Check sheet for the modelled part. Datum: model origin and axes. Units: mm. A direction names the side the tool comes from. Round coordinates to 2 decimals unless told otherwise and drop trailing zeros. Write each loop counter-clockwise with the first axis right and the second up, starting at its lowest first coordinate (ties: lowest second). Pieces come first, ordered by that corner, then holes. Notation, with made-up numbers: M -29.5,44.25 L 1.5,44.25 A14 cw 1.5,56.25 Z; hole C 73.5,31 d9. An arc over 180 degrees is marked long. Put each result on its own line as item: value.
```python
from build123d import *

# Parameters (mm, degrees)
F0_R     = 9.085858
F0_R_2   = 9.713119
F0_R_3   = 9.943087
F1_DEPTH = 20
F0_R_4   = 2.956613
F0_R_5   = 3.792216
F0_R_6   = 3.328406
F2_DEPTH = 10


with BuildPart() as f1:
    # F0 (on Top) → F1 (new body)
    with BuildSketch(Plane.XY):
        with BuildLine():
            ThreePointArc((0, 16), (4.686292, 4.686292), (16, 0))
            Line((16, 0), (62.072559, 0))
            ThreePointArc((62.072559, 0), (77.309287, 11.117161), (71.37237, 29.019736))
            Line((71.37237, 29.019736), (25.299811, 61.928706))
            ThreePointArc((25.299811, 61.928706), (8.678695, 63.135653), (0, 48.908971))
            Line((0, 48.908971), (0, 16))
        make_face()
        with Locations((16, 16)):
            Circle(F0_R, mode=Mode.SUBTRACT)
        with Locations((62.072559, 16)):
            Circle(F0_R_2, mode=Mode.SUBTRACT)
        with Locations((16, 48.908971)):
            Circle(F0_R_3, mode=Mode.SUBTRACT)
    extrude(amount=F1_DEPTH)

    # F0 (on Top) → F2 (join)
    with BuildSketch(Plane.XY):
        with Locations((16, 16)):
            Circle(F0_R)
        with Locations((16, 16)):
            Circle(F0_R_4, mode=Mode.SUBTRACT)
        with Locations((16, 48.908971)):
            Circle(F0_R_3)
        with Locations((16, 48.908971)):
            Circle(F0_R_5, mode=Mode.SUBTRACT)
        with Locations((62.072559, 16)):
            Circle(F0_R_2)
        with Locations((62.072559, 16)):
            Circle(F0_R_6, mode=Mode.SUBTRACT)
    extrude(amount=F2_DEPTH)


solid = f1.part
```
1. Release check for a two-part mould opening along X. For faces 1 (the cylindrical face through (6.923, 16.399, 14.93)), 2 (the flat face through (30, 26, 0)), 3 (the cylindrical face through (77.22, 10.85, 9.86)), 4 (the flat face through (20, 16, 10)) record: +X half, -X half, draft (parallel to the pull), parting line (faces both ways), or undercut.
Computed values:
face 1: undercut
face 2: draft
face 3: +X half
face 4: undercut
2. Cross-section at C-C (y = 9). Enter the section's corners in (x, z).
Computed values:
outline: M 1.61,0 L 76.46,0 L 76.46,20 L 68.81,20 L 68.81,10 L 55.34,10 L 55.34,20 L 21.79,20 L 21.79,10 L 10.21,10 L 10.21,20 L 1.61,20 Z
3. Depth check by flat-ended pin: pin 1 Ø3 at (x, y) = (59.5, 32.5) entering from -Z; pin 2 Ø5.5 at (x, y) = (62.07, 16) entering from -Z; pin 3 Ø4 at (x, z) = (44.5, 6) entering from +Y; pin 4 Ø16 at (x, y) = (16, 50) entering from +Z. Enter the tip coordinate at first touch or a pass-through.
Computed values:
pin 1: stops at z = 0
pin 2: passes through
pin 3: stops at y = 49.64
pin 4: stops at z = 10
4. Access from +Z, -Z, +X, -X, +Y, -Y to the whole of each face (thin tool, end or side, straight path). Record for faces 5 (the cylindrical face through (67.294, 24.19, 14.93)), 6 (the cylindrical face through (4.563, 4.811, 9.86)).
Computed values:
face 5: +Z
face 6: +Z, -Z, -X, -Y
5. Cross-section at B-B (x = 17). Enter the section's corners in (y, z).
Computed values:
outline: M 0,0 L 13.22,0 L 13.22,10 L 6.97,10 L 6.97,20 L 0,20 Z; M 18.78,0 L 45.25,0 L 45.25,10 L 39.02,10 L 39.02,20 L 25.03,20 L 25.03,10 L 18.78,10 Z; M 52.57,0 L 64.88,0 L 64.88,20 L 58.8,20 L 58.8,10 L 52.57,10 Z
6. Cross-section at A-A (z = 7.25). Enter the section's corners in (x, y).
Computed values:
outline: M 0,16 A16 ccw 16,0 L 62.07,0 A16 ccw 71.37,29.02 L 25.3,61.93 A16 ccw 0,48.91 Z; hole C 16,48.91 d7.58; hole C 16,16 d5.91; hole C 62.07,16 d6.66
7. Cross-section at D-D (z = 14.5). Enter the section's corners in (x, y).
Computed values:
outline: M 0,16 A16 ccw 16,0 L 62.07,0 A16 ccw 71.37,29.02 L 25.3,61.93 A16 ccw 0,48.91 Z; hole C 16,48.91 d19.89; hole C 16,16 d18.17; hole C 62.07,16 d19.43
8. Scan lines: probe 1 along X at (y, z) = (17.5, 12); probe 2 along Z at (x, y) = (17.5, 22); probe 3 along X at (y, z) = (20, 10.5). Record each from-to range of solid material in increasing order.
Computed values:
probe 1: x = 0 to 7.04, 24.96 to 52.48, 71.67 to 78
probe 2: z = 0 to 10
probe 3: x = 0 to 7.84, 24.16 to 53.22, 70.92 to 77.56
